from build123d import *

# Parameters (mm, degrees)
SKETCH1_W            = 31.2
SKETCH1_H            = 26.2
BOSS_EXTRUDE1_DEPTH  = 15
SHELL2_T             = -3
BOSS_EXTRUDE2_DEPTH  = 10
CUT_EXTRUDE2_DEPTH   = 43.175822458
SKETCH8_R            = 2.15
BOSS_EXTRUDE5_DEPTH  = 3
CUT_EXTRUDE7_DEPTH   = 1
SKETCH14_W           = 25.2
SKETCH14_H           = 20.2
CUT_EXTRUDE5_DEPTH   = 36.815778646
BOSS_EXTRUDE8_REACH  = 45.959
BOSS_EXTRUDE9_START  = -8
SKETCH15_W           = 31.2
SKETCH15_H           = 26.2
SKETCH15_W_2         = 14.5
SKETCH15_H_2         = 17
BOSS_EXTRUDE9_DEPTH  = 2
SKETCH16_R           = 2.4
SKETCH16_R_2         = 1.4
BOSS_EXTRUDE10_DEPTH = 4.41
CUT_EXTRUDE6_REACH   = 48.267
SKETCH5_W            = 10
SKETCH5_H            = 4.18


with BuildPart() as part:
    # Sketch1 → Boss-Extrude1 (new body)
    with BuildSketch(Plane.XY):
        Rectangle(SKETCH1_W, SKETCH1_H)
    extrude(amount=BOSS_EXTRUDE1_DEPTH)

    # Shell2
    shell2_openings = [part.faces().sort_by_distance(p)[0] for p in [
        (0, 0, 0),
    ]]
    offset(amount=SHELL2_T, openings=shell2_openings, kind=Kind.INTERSECTION)

    # Sketch3 → Boss-Extrude2 (add)
    with BuildSketch(Plane(origin=(0, 13.1, 0), x_dir=(1, 0, 0), z_dir=(0, 1, 0))):
        with BuildLine():
            Line((-6, 0), (-3, 0))
            ThreePointArc((-3, 0), (0, -3), (3, 0))
            Line((3, 0), (6, 0))
            ThreePointArc((6, 0), (0, -6), (-6, 0))
        make_face()
    boss_extrude2 = extrude(amount=BOSS_EXTRUDE2_DEPTH)

    # Mirror1: Boss-Extrude2 across plane
    add(boss_extrude2.mirror(Plane.ZX))

    # Sketch4 → Cut-Extrude2 (cut, through all)
    with BuildSketch(Plane(origin=(0, 13.1, 0), x_dir=(1, 0, 0), z_dir=(0, 1, 0))):
        with BuildLine():
            Line((-3, 0), (3, 0))
            ThreePointArc((3, 0), (0, -3), (-3, 0))
        make_face()
    extrude(amount=-CUT_EXTRUDE2_DEPTH, mode=Mode.SUBTRACT)

    # Sketch8 → Boss-Extrude5 (add)
    # profile 1 of 2: a face of its own
    with BuildSketch(Plane(origin=(0, 0, 0), x_dir=(-1, 0, 0), z_dir=(0, 0, -1))):
        with BuildLine():
            Line((-15.6, 3), (-15.6, 11))
            Line((-15.6, 11), (-20.6, 11))
            ThreePointArc((-20.6, 11), (-24.6, 7), (-20.6, 3))
            Line((-20.6, 3), (-15.6, 3))
        make_face()
        with Locations((-20.6, 7)):
            Circle(SKETCH8_R, mode=Mode.SUBTRACT)
    # profile 2 of 2: a face of its own
    with BuildSketch(Plane(origin=(0, 0, 0), x_dir=(-1, 0, 0), z_dir=(0, 0, -1))):
        with BuildLine():
            Line((-15.6, -11), (-15.6, -3))
            Line((-15.6, -3), (-20.6, -3))
            ThreePointArc((-20.6, -3), (-24.6, -7), (-20.6, -11))
            Line((-20.6, -11), (-15.6, -11))
        make_face()
        with Locations((-20.6, -7)):
            Circle(SKETCH8_R, mode=Mode.SUBTRACT)
    boss_extrude5 = extrude(amount=-BOSS_EXTRUDE5_DEPTH)

    # Sketch7 → Cut-Extrude7 (cut)
    with BuildSketch(Plane(origin=(0, 0, 0), x_dir=(-1, 0, 0), z_dir=(0, 0, -1))):
        Polygon((-3.85, -23.1), (-3.85, -10.95), (-13.45, -10.95), (-13.45, 10.95), (-3.85, 10.95), (-3.85, 23.1), (-5.15, 23.1), (-5.15, 12.25), (-14.75, 12.25), (-14.75, -12.25), (-5.15, -12.25), (-5.15, -23.1), align=None)
    cut_extrude7 = extrude(amount=-CUT_EXTRUDE7_DEPTH, mode=Mode.SUBTRACT)

    # Mirror3: Boss-Extrude5, Cut-Extrude7 across plane
    add(boss_extrude5.mirror(Plane(origin=(0, 0, 0), x_dir=(0, 0, 1), z_dir=(1, 0, 0))))
    add(cut_extrude7.mirror(Plane(origin=(0, 0, 0), x_dir=(0, 0, 1), z_dir=(1, 0, 0))), mode=Mode.SUBTRACT)

    # Sketch14 → Cut-Extrude5 (cut, through all)
    with BuildSketch(Plane(origin=(0, 0, 12), x_dir=(-1, 0, 0), z_dir=(0, 0, -1))):
        Rectangle(SKETCH14_W, SKETCH14_H)
    extrude(amount=-CUT_EXTRUDE5_DEPTH, mode=Mode.SUBTRACT)

    # Sketch11 → Boss-Extrude8 (add, up to next)
    with BuildSketch(Plane(origin=(0, -10.1, 0), x_dir=(1, 0, 0), z_dir=(0, 1, 0)), mode=Mode.PRIVATE) as boss_extrude8_sk1:
        with BuildLine():
            Line((3, 0), (12.6, 0))
            Line((12.6, 0), (12.6, -5.002969955))
            Line((12.6, -5.002969955), (2.801311304, -1.073617705))
            ThreePointArc((2.801311304, -1.073617705), (2.949909652, -0.545924027), (3, 0))
        make_face()
    boss_extrude8_tool1 = extrude(boss_extrude8_sk1.sketch, amount=BOSS_EXTRUDE8_REACH, mode=Mode.PRIVATE) - part.part
    # Sketch11 → Boss-Extrude8 (add, up to next)
    with BuildSketch(Plane(origin=(0, -10.1, 0), x_dir=(1, 0, 0), z_dir=(0, 1, 0)), mode=Mode.PRIVATE) as boss_extrude8_sk2:
        with BuildLine():
            Line((-12.6, -5.002969955), (-2.801311304, -1.073617705))
            ThreePointArc((-2.801311304, -1.073617705), (-2.949909652, -0.545924027), (-3, 0))
            Line((-3, 0), (-12.6, 0))
            Line((-12.6, 0), (-12.6, -5.002969955))
        make_face()
    boss_extrude8_tool2 = extrude(boss_extrude8_sk2.sketch, amount=BOSS_EXTRUDE8_REACH, mode=Mode.PRIVATE) - part.part
    add(boss_extrude8_tool1.solids().sort_by_distance((8.785084, -10.1, 1.737296))[0])
    add(boss_extrude8_tool2.solids().sort_by_distance((-8.785084, -10.1, 1.737296))[0])

    # Sketch15 → Boss-Extrude9 (add)
    with BuildSketch(Plane.XY.offset(15).offset(BOSS_EXTRUDE9_START)):
        Rectangle(SKETCH15_W, SKETCH15_H)
        Rectangle(SKETCH15_W_2, SKETCH15_H_2, mode=Mode.SUBTRACT)
    extrude(amount=BOSS_EXTRUDE9_DEPTH)

    # Sketch16 → Boss-Extrude10 (add)
    # profile 1 of 4: a face of its own
    with BuildSketch(Plane.XY.offset(9)):
        with Locations((-10, 7.5)):
            Circle(SKETCH16_R)
        with Locations((-10, 7.5)):
            Circle(SKETCH16_R_2, mode=Mode.SUBTRACT)
    # profile 2 of 4: a face of its own
    with BuildSketch(Plane.XY.offset(9)):
        with Locations((10, 7.5)):
            Circle(SKETCH16_R)
        with Locations((10, 7.5)):
            Circle(SKETCH16_R_2, mode=Mode.SUBTRACT)
    # profile 3 of 4: a face of its own
    with BuildSketch(Plane.XY.offset(9)):
        with Locations((-10, -7.5)):
            Circle(SKETCH16_R)
        with Locations((-10, -7.5)):
            Circle(SKETCH16_R_2, mode=Mode.SUBTRACT)
    # profile 4 of 4: a face of its own
    with BuildSketch(Plane.XY.offset(9)):
        with Locations((10, -7.5)):
            Circle(SKETCH16_R)
        with Locations((10, -7.5)):
            Circle(SKETCH16_R_2, mode=Mode.SUBTRACT)
    extrude(amount=BOSS_EXTRUDE10_DEPTH)

    # Sketch5 → Cut-Extrude6 (cut, up to next)
    with BuildSketch(Plane(origin=(0, 13.1, 0), x_dir=(1, 0, 0), z_dir=(0, 1, 0)), mode=Mode.PRIVATE) as cut_extrude6_sk1:
        with Locations((0, -11.31)):
            Rectangle(SKETCH5_W, SKETCH5_H)
    cut_extrude6_tool1 = extrude(cut_extrude6_sk1.sketch, amount=-CUT_EXTRUDE6_REACH, mode=Mode.PRIVATE) & part.part
    add(cut_extrude6_tool1.solids().sort_by_distance((0, 13.1, 11.31))[0], mode=Mode.SUBTRACT)


solid = part.part
The listing builds one solid part. Answer for the finished solid, in the listing's coordinates (mm). A direction names the side the tool comes from. Round coordinates to 2 decimals unless told otherwise and drop trailing zeros. Order: outer loops, then holes, each group sorted by start corner. A loop starts at its lowest first (then second) coordinate and runs counter-clockwise, first axis right, second up. Notation, with made-up numbers: (61.5, 9) -> (85.5, 9) arc R26 cw to (85.5, 48) -> close; hole circle Ø5 at (31.5, 45). An arc over 180 degrees is marked (long way). Write each question's results on one line, items separated by ' | '. Start each with the question number.
Q1. The mould has two halves that part along Z. Classify faces 5 (the flat face through (-18, -7, 3)), 6 (the flat face through (-7.769, -0.141, 3.066)), 7 (the flat face through (0, -23.1, 4)): pulls with the +Z half, pulls with the -Z half, needs draft (parallel to the pull), parting line crosses it, or undercut.
Q2. Which of the six approach directions +Z, -Z, +X, -X, +Y, -Y give full straight-line access (tool end or side, diameter ignored) to faces 1 (the flat face through (0, -10.1, 5)), 2 (the flat face through (18, 3, 1)), 3 (the flat face through (-5, 12, 11)), 4 (the flat face through (0, -10.1, 12))?
Q3. Straight lines are drawn through the part: probe 1 along Y at (x, z) = (20.6, 1.2); probe 2 along Y at (x, z) = (-10, 11.35); probe 3 along Y at (x, z) = (-12.5, 13). For each, find the intervals that lie inside material, in ascending order. Write a range as from..to.
Q4. Each of these flat-tipped pins is pushed along its axis until it touches: pin 1 (5 mm diameter, centred on y = -3.5, z = 7.5, fed in from -X); pin 2 (0.8 mm diameter, centred on x = 9.5, z = 0.5, fed in from +Y); pin 3 (5 mm diameter, centred on x = 5.5, z = 12.5, fed in from -Y). Where does it stop, or does it pass through?
Q5. Find section C-C (y = 15.5). Determine the outline of the cut face in (x, z), then the cut area to 3 significant figures.
Q6. Find section A-A (x = 0). Determine the outline of the cut face in (y, z), then the cut area to 3 significant figures.
Q7. Find section B-B (y = 1). Determine the outline of the cut face in (x, z).
Worked answers:
1) face 5: pulls with the +Z half | face 6: undercut | face 7: needs draft
2) face 1: none | face 2: +Z, -Z, +X | face 3: +Y | face 4: +Z
3) probe 1: y = -11..-9.15, -4.85..-3, 3..4.85, 9.15..11 | probe 2: y = -13.1..-10.1, -9.9..-8.9, -6.1..-5.1, 5.1..6.1, 8.9..9.9, 10.1..13.1 | probe 3: y = -13.1..-10.1, 10.1..13.1
4) pin 1: stops at x = -15.6 | pin 2: stops at y = 13.1 | pin 3: stops at y = -13.1
5) outline: (-6, 0) -> (-5.15, 0) -> (-5.15, 1) -> (-3.85, 1) -> (-3.85, 0) -> (-3, 0) arc R3 cw to (3, 0) -> (3.85, 0) -> (3.85, 1) -> (5.15, 1) -> (5.15, 0) -> (6, 0) arc R6 ccw to start | area: 39.8 mm2
6) outline: (-23.1, 3) -> (-10.1, 3) -> (-10.1, 7) -> (-8.5, 7) -> (-8.5, 9) -> (-10.1, 9) -> (-10.1, 15) -> (-13.1, 15) -> (-13.1, 6) -> (-23.1, 6) -> close; (8.5, 7) -> (10.1, 7) -> (10.1, 3) -> (23.1, 3) -> (23.1, 6) -> (13.1, 6) -> (13.1, 9.22) -> (10.1, 9.22) -> (10.1, 9) -> (8.5, 9) -> close; (10.1, 13.4) -> (13.1, 13.4) -> (13.1, 15) -> (10.1, 15) -> close | area: 126 mm2
7) outline: (-15.6, 0) -> (-14.75, 0) -> (-14.75, 1) -> (-13.45, 1) -> (-13.45, 0) -> (-3, 0) arc R3 cw to (-2.8, 1.07) -> (-12.6, 5) -> (-12.6, 7) -> (-7.25, 7) -> (-7.25, 9) -> (-12.6, 9) -> (-12.6, 15) -> (-15.6, 15) -> close; (2.8, 1.07) arc R3 cw to (3, 0) -> (13.45, 0) -> (13.45, 1) -> (14.75, 1) -> (14.75, 0) -> (15.6, 0) -> (15.6, 15) -> (12.6, 15) -> (12.6, 9) -> (7.25, 9) -> (7.25, 7) -> (12.6, 7) -> (12.6, 5) -> close
